Can you work these out from the drawing? Everything is in mm from the part's minimum corner. Round coordinates to 2 decimals unless told otherwise and drop trailing zeros. Write each question's results on one line, items separated by ' | '. Start each with the question number.
(1) Please list where these lines run through material, in increasing order: line 1 (Z direction, x = 307, y = 2.75); line 2 (X direction, y = 5.75, z = 7.75); line 3 (X direction, y = 1.5, z = 9.5). Write a range as [from, to].
(2) For P1, Ø3, axis at y = 5, z = 9, coming from the +X side; P2, Ø3, axis at y = 2, z = 10, coming from the -X side, each with a flat end and sliding along its axis, tell me the tip position at first contact or that it passes through.
(3) Imagine slicing it at A-A on y = 3.75. State how many separate pieces and enclosed holes the cut face has, then the cut area to 3 significant figures.
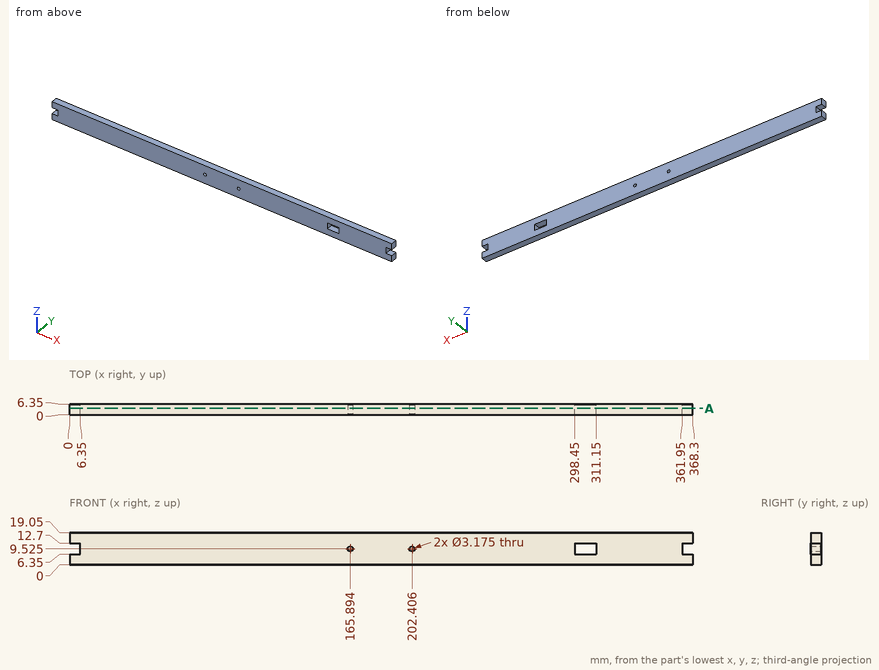
Response:
1) line 1: [0, 6.35], [12.7, 19.05] | line 2: [6.35, 298.45], [311.15, 361.95] | line 3: [6.35, 164.31], [167.48, 200.82], [203.99, 298.45], [311.15, 361.95]
2) P1: x = 361.95 | P2: x = 6.35
3) separate pieces: 1 | enclosed holes: 3 | area: 6,840 mm²
